```python
from build123d import *

# Parameters (mm, degrees)
SKETCH1_R                  = 35
EXTRUDE1_DEPTH             = 25
EXTRUDE1_DRAFT             = -15
SKETCH2_R                  = 8
EXTRUDE2_DEPTH             = 12
SKETCH3_W                  = 10
SKETCH3_H                  = 30
CUT_EXTRUDE1_DEPTH         = 70.617297676
EXTRUDE4_DEPTH             = 1
F_11_0_11_DIAMETER_HOLE1_D = 11


with BuildPart() as part:
    # Sketch1 → Extrude1 (with draft: the straight prism first)
    with BuildSketch(Plane(origin=(0, 0, 0), x_dir=(1, 0, 0), z_dir=(0, 1, 0))):
        Circle(SKETCH1_R)
    extrude(amount=EXTRUDE1_DEPTH)
    # Extrude1: the draft: its side faces are tilted about the plane it starts from
    extrude1_sides = [part.faces().sort_by_distance(p)[0] for p in [
        (-35, 12.5, 0),
    ]]
    draft(extrude1_sides, Plane(origin=(0, 0, 0), x_dir=(1, 0, 0), z_dir=(0, 1, 0)), EXTRUDE1_DRAFT)

    # Sketch2 → Extrude2 (add)
    with BuildSketch(Plane.XZ):
        with Locations(Location((0, 0, 0), (0, 0, 90))):
            Circle(SKETCH2_R)
    extrude(amount=EXTRUDE2_DEPTH)

    # Sketch3 → Cut-Extrude1 (cut, through all)
    with BuildSketch(Plane(origin=(0, 25, 0), x_dir=(1, 0, 0), z_dir=(0, 1, 0))):
        with Locations((0, 40)):
            Rectangle(SKETCH3_W, SKETCH3_H)
    extrude(amount=-CUT_EXTRUDE1_DEPTH, mode=Mode.SUBTRACT)

    # Sketch5 → Extrude4 (add)
    with BuildSketch(Plane(origin=(0, 25, 0), x_dir=(1, 0, 0), z_dir=(0, 1, 0))):
        with BuildLine():
            Line((-5, 25), (-5, 41.397875161))
            ThreePointArc((-5, 41.397875161), (0, -41.698729811), (5, 41.397875161))
            Line((5, 41.397875161), (5, 25))
            Line((5, 25), (-5, 25))
        make_face()
    extrude(amount=EXTRUDE4_DEPTH)

    # Ø11.0 (11) Diameter Hole1 (through all)
    with Locations(Plane(origin=(0, 26, 0), x_dir=(1, 0, 0), z_dir=(0, 1, 0))):
        with Locations((0, 0)):
            Hole(F_11_0_11_DIAMETER_HOLE1_D / 2)


solid = part.part
```
Here's how the part is built. I have some questions about the finished solid (model axes, mm). A direction names the side the tool comes from. Round coordinates to 2 decimals unless told otherwise and drop trailing zeros. Loops run counter-clockwise (first coordinate to the right, second up) from the corner with the lowest first, then second, coordinate; pieces in that order, holes last.
1. For faces 1 (the face through (7.81, -5.92, -1.73)), 2 (the face through (1.19, 6.73, 5.37)), 3 (the face through (0, 13, -25)), which set-ups out of +Z, -Z, +X, -X, +Y, -Y let a thin tool reach every point of the face, with its end or its side?
Answers:
face 1: -Y
face 2: +Y, -Y
face 3: -Z, +Y, -Y
2. Suppose I cut it at B-B, the plane z = 0. Please give me the cut outline in (x, y), and give its area (3 significant figures).
Answers:
outline: (-41.7, 25) - (-35, 0) - (-8, 0) - (-8, -12) - (-5.5, -12) - (-5.5, 26) - (-41.7, 26) - close; (5.5, -12) - (8, -12) - (8, 0) - (35, 0) - (41.7, 25) - (41.7, 26) - (5.5, 26) - close
area: 1,770 mm2
3. If I drill on probe 1 along Y at (x, z) = (-25.5, 20); probe 2 along Z at (x, y) = (-0.5, -4); probe 3 along Z at (x, y) = (3.5, -0.5), over which ranges is the centre line in solid material (lowest first)?
Answers:
probe 1: y = 0 to 26
probe 2: z = -7.98 to -5.48, 5.48 to 7.98
probe 3: z = -7.19 to -4.24, 4.24 to 7.19
4. Suppose I cut it at D-D, the plane y = -1. Please give me the cut outline in (x, z).
Answers:
outline: circle Ø16 at (0, 0); hole circle Ø11 at (0, 0)
5. Suppose I cut it at A-A, the plane x = 0. Please give me the cut outline in (y, z).
Answers:
outline: (-12, -8) - (0, -8) - (0, -25) - (26, -25) - (26, -5.5) - (-12, -5.5) - close; (-12, 5.5) - (26, 5.5) - (26, 41.7) - (25, 41.7) - (0, 35) - (0, 8) - (-12, 8) - close
6. Will these pins go through, and if not, where does the flat tip stop? pin 1 (1.5 mm diameter, centred on y = 15, z = 6.5, fed in from -X); pin 2 (12 mm diameter, centred on y = -6.5, z = -4.5, fed in from +X); pin 3 (5 mm diameter, centred on x = 20, y = 1, fed in from +Z).
Answers:
pin 1: stops at x = -38.71
pin 2: stops at x = 8
pin 3: stops at z = 30.81
7. Suppose I cut it at C-C, the plane y = 8. Please give me the cut outline in (x, z), and give its area (3 significant figures).
Answers:
outline: (-5, -36.81) - (-5, -25) - (5, -25) - (5, -36.81) arc R37.14 ccw (long way) to start; hole circle Ø11 at (0, 0)
area: 4,120 mm2
